Geometry check sheet. Reference: the model listing, model coordinates, mm. Face numbers are marked on the shaded views. A direction names the side the tool comes from. Coordinates: 2 decimals unless noted, no trailing zeros. Write each loop counter-clockwise with the first axis right and the second up, starting at its lowest first coordinate (ties: lowest second). Pieces come first, ordered by that corner, then holes. Notation, with made-up numbers: (-35.5, 14) -> (-31.5, 14) arc R24 cw to (-31.5, 24) -> close; hole circle Ø5 at (-21.5, -24.75). An arc over 180 degrees is marked (long way). Put each result on its own line as item: value. Start each with the question number.
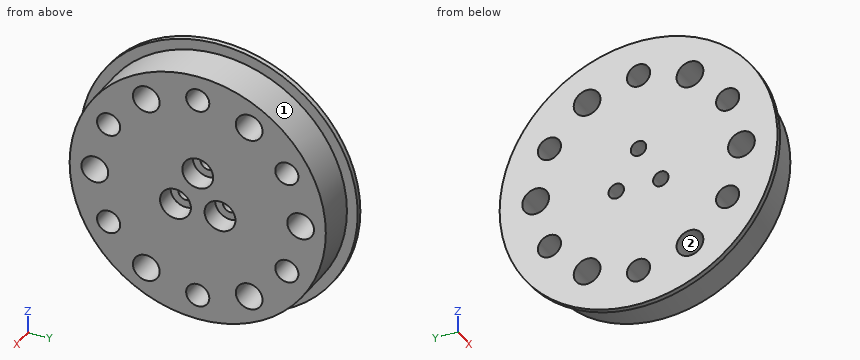
from build123d import *

# Parameters (mm, degrees)
SKETCH020_R     = 27
SKETCH020_R_2   = 1.5
SKETCH020_R_3   = 2.25
SKETCH020_R_4   = 2.6
PAD017_DEPTH    = 9
SKETCH021_R     = 30
SKETCH021_R_2   = 24.9
POCKET003_DEPTH = 8
SKETCH022_R     = 3
POCKET004_DEPTH = 4


with BuildPart() as part:
    # Sketch020 → Pad017 (new body)
    with BuildSketch(Plane.YZ):
        Circle(SKETCH020_R)
        with Locations((0, 5)):
            Circle(SKETCH020_R_2, mode=Mode.SUBTRACT)
        with Locations((-4.330127, -2.5)):
            Circle(SKETCH020_R_2, mode=Mode.SUBTRACT)
        with Locations((4.330127, -2.5)):
            Circle(SKETCH020_R_2, mode=Mode.SUBTRACT)
        with Locations((0, 20)):
            Circle(SKETCH020_R_3, mode=Mode.SUBTRACT)
        with Locations((0, -20)):
            Circle(SKETCH020_R_3, mode=Mode.SUBTRACT)
        with Locations((17.320508, -10)):
            Circle(SKETCH020_R_3, mode=Mode.SUBTRACT)
        with Locations((-17.320508, -10)):
            Circle(SKETCH020_R_3, mode=Mode.SUBTRACT)
        with Locations((-17.320508, 10)):
            Circle(SKETCH020_R_3, mode=Mode.SUBTRACT)
        with Locations((17.320508, 10)):
            Circle(SKETCH020_R_3, mode=Mode.SUBTRACT)
        with Locations((20, 0)):
            Circle(SKETCH020_R_4, mode=Mode.SUBTRACT)
        with Locations((-20, 0)):
            Circle(SKETCH020_R_4, mode=Mode.SUBTRACT)
        with Locations((-10, -17.320508)):
            Circle(SKETCH020_R_4, mode=Mode.SUBTRACT)
        with Locations((10, -17.320508)):
            Circle(SKETCH020_R_4, mode=Mode.SUBTRACT)
        with Locations((10, 17.320508)):
            Circle(SKETCH020_R_4, mode=Mode.SUBTRACT)
        with Locations((-10, 17.320508)):
            Circle(SKETCH020_R_4, mode=Mode.SUBTRACT)
    extrude(amount=PAD017_DEPTH)

    # Sketch021 (on DatumPlane) → Pocket003 (cut)
    with BuildSketch(Plane.YZ.offset(9)):
        Circle(SKETCH021_R)
        Circle(SKETCH021_R_2, mode=Mode.SUBTRACT)
    extrude(amount=-POCKET003_DEPTH, mode=Mode.SUBTRACT)

    # Sketch022 (on DatumPlane) → Pocket004 (cut)
    with BuildSketch(Plane.YZ.offset(9)):
        with Locations((0, 5)):
            Circle(SKETCH022_R)
        with Locations((4.330127, -2.5)):
            Circle(SKETCH022_R)
        with Locations((-4.330127, -2.5)):
            Circle(SKETCH022_R)
    extrude(amount=-POCKET004_DEPTH, mode=Mode.SUBTRACT)


solid = part.part
Item 1: Go/stop test with flat-tipped pins: P1, Ø2, axis at x = 2.5, z = -17.5, coming from the +Y side; P2, Ø1.8, axis at y = -3, z = -3.5, coming from the +X side; P3, Ø4.5, axis at y = -10, z = 17.32, coming from the -X side; P4, Ø1.5, axis at x = 3.5, z = 3, coming from the -Y side. Record where each tip stops, or that it passes through.
Item 2: Section check B-B, the plane z = 10. Enter the section's corners in (x, y), and give its area (3 significant figures).
Item 3: Access from +Z, -Z, +X, -X, +Y, -Y to the whole of each face (thin tool, end or side, straight path). Record for the marked faces 1 and 2.
Item 4: Section check D-D, the plane y = -10. Enter the section's corners in (x, z).
Item 5: Scan lines: line 1 along Z through (x, y) = (6.5, 0); line 2 along Z through (x, y) = (5, -10); line 3 along Z through (x, y) = (6.5, -8.5). Record each from-to range of solid material in increasing order. Write a range as [from, to].
Item 6: Section check C-C, the plane x = 7.25. Give the number of separate pieces and of enclosed holes in the cut face, and give its area (3 significant figures).
Item 7: Section check A-A, the plane y = 0. Enter the section's corners in (x, z).
From the geometry:
1. P1: y = 18.65
1. P2: x = 5
1. P3: through
1. P4: y = -24.8
2. outline: (0, -25.08) -> (1, -25.08) -> (1, -22.8) -> (9, -22.8) -> (9, -19.57) -> (0, -19.57) -> close; (0, -15.07) -> (9, -15.07) -> (9, 15.07) -> (0, 15.07) -> close; (0, 19.57) -> (9, 19.57) -> (9, 22.8) -> (1, 22.8) -> (1, 25.08) -> (0, 25.08) -> close
2. area: 334 mm²
3. face 1: +X
3. face 2: +X, -X
4. outline: (0, -25.08) -> (1, -25.08) -> (1, -22.8) -> (9, -22.8) -> (9, -19.92) -> (0, -19.92) -> close; (0, -14.72) -> (9, -14.72) -> (9, 14.72) -> (0, 14.72) -> close; (0, 19.92) -> (9, 19.92) -> (9, 22.8) -> (1, 22.8) -> (1, 25.08) -> (0, 25.08) -> close
5. line 1: [-24.9, -22.25], [-17.75, 2], [8, 17.75], [22.25, 24.9]
5. line 2: [-22.8, -19.92], [-14.72, 14.72], [19.92, 22.8]
5. line 3: [-23.4, -19.44], [-15.2, 15.2], [19.44, 23.4]
6. separate pieces: 1
6. enclosed holes: 15
6. area: 1,640 mm²
7. outline: (0, -27) -> (1, -27) -> (1, -24.9) -> (9, -24.9) -> (9, -22.25) -> (0, -22.25) -> close; (0, -17.75) -> (9, -17.75) -> (9, 2) -> (5, 2) -> (5, 3.5) -> (0, 3.5) -> close; (0, 6.5) -> (5, 6.5) -> (5, 8) -> (9, 8) -> (9, 17.75) -> (0, 17.75) -> close; (0, 22.25) -> (9, 22.25) -> (9, 24.9) -> (1, 24.9) -> (1, 27) -> (0, 27) -> close
